```python
from build123d import *

# Parameters (mm, degrees)
BOSS_EXTRUDE1_DEPTH = 4.7625
SKETCH3_W           = 66.200858932
SKETCH3_H           = 5.079818348
BOSS_EXTRUDE2_DEPTH = 31.75
SKETCH4_W           = 28.999942
SKETCH4_H           = 12.9999994
CUT_EXTRUDE1_DEPTH  = 4.7625
SKETCH5_R           = 6.4999997
CUT_EXTRUDE2_DEPTH  = 4.7625
SKETCH6_R           = 3.175
CUT_EXTRUDE3_DEPTH  = 7.3025


with BuildPart() as part:
    # Sketch1 → Boss-Extrude1 (new body)
    with BuildSketch(Plane.XY):
        Polygon((30.222809818, 36.11360466), (25.142809818, 48.349181892), (-47.247190182, 48.349181892), (-52.327190182, 36.11360466), (-52.327190182, -53.715240876), (-47.247190182, -65.950818108), (25.142809818, -65.950818108), (30.222809818, -53.715240876), align=None)
    extrude(amount=BOSS_EXTRUDE1_DEPTH)

    # Sketch3 → Boss-Extrude2 (add)
    with BuildSketch(Plane.XY.offset(4.7625)):
        with Locations((-11.098760716, 45.809272718)):
            Rectangle(SKETCH3_W, SKETCH3_H)
        with Locations((-11.098760716, -63.410908934)):
            Rectangle(SKETCH3_W, SKETCH3_H)
    extrude(amount=BOSS_EXTRUDE2_DEPTH)

    # Sketch4 → Cut-Extrude1 (cut)
    with BuildSketch(Plane(origin=(0, 0, 0), x_dir=(-1, 0, 0), z_dir=(0, 0, -1))):
        with Locations((11.052190182, -27.850818108)):
            Rectangle(SKETCH4_W, SKETCH4_H)
    extrude(amount=-CUT_EXTRUDE1_DEPTH, mode=Mode.SUBTRACT)

    # Sketch5 → Cut-Extrude2 (cut)
    with BuildSketch(Plane(origin=(0, 0, 0), x_dir=(-1, 0, 0), z_dir=(0, 0, -1))):
        with Locations((11.052190182, 10.249181892)):
            Circle(SKETCH5_R)
    extrude(amount=-CUT_EXTRUDE2_DEPTH, mode=Mode.SUBTRACT)

    # Sketch6 → Cut-Extrude3 (cut)
    with BuildSketch(Plane.XZ.offset(65.950818108)):
        with Locations((-11.052190182, 20.6375)):
            Circle(SKETCH6_R)
    extrude(amount=-CUT_EXTRUDE3_DEPTH, mode=Mode.SUBTRACT)


solid = part.part
```
Verification items for the finished model (mm, model axes). A direction names the side the tool comes from. Give positions to 0.01 mm unless a question says otherwise; leave off trailing zeros. Loops run counter-clockwise (first coordinate to the right, second up) from the corner with the lowest first, then second, coordinate; pieces in that order, holes last.
1. Section check B-B, the plane z = 10. Enter the section's corners in (x, y).
2. Set-up check for faces 1 (the flat face through (-12, -60.871, 24)), 2 (the flat face through (-11, -34.351, 2)), 3 (the flat face through (22.002, -63, 20)), 4 (the flat face through (-44.199, -63, 20)): record each of +Z, -Z, +X, -X, +Y, -Y from which the full face is reachable in a straight line by a thin tool's end or side.
3. Go/stop test with flat-tipped pins: pin 1 Ø15 at (x, y) = (-11.05, 10.25) entering from +Z; pin 2 Ø2.5 at (y, z) = (46, 27) entering from +X; pin 3 Ø1.5 at (y, z) = (46, 25.5) entering from -X. Record where each tip stops, or that it passes through.
4. Thickness scan on line 1 (Y direction, x = 17.5, z = 20); line 2 (X direction, y = -28, z = 2); line 3 (Z direction, x = -45, y = -50.5). Record the ranges inside material, lowest first.
5. Section check D-D, the plane x = 8. Enter the section's corners in (y, z).
6. Section check A-A, the plane y = -27. Enter the section's corners in (x, z), then the cut area to 3 significant figures.
7. Mould release check, pull along Z, two halves, no side actions. Record for faces 5 (the flat face through (-12, 43.269, 20)), 6 (the flat face through (-12, -8, 0)), 7 (the cylindrical face through (-14.224, -63.446, 20.777)), 8 (the flat face through (-12, 46, 36.512)): released by +Z, released by -Z, zero draft, split by the parting line, or undercut.
8. Section check C-C, the plane z = 22.5. Enter the section's corners in (x, y), then the cut area to 3 significant figures.
Geometry says:
1. outline: (-44.2, -65.95) - (22, -65.95) - (22, -60.87) - (-44.2, -60.87) - close; (-44.2, 43.27) - (22, 43.27) - (22, 48.35) - (-44.2, 48.35) - close
2. face 1: +Z, +X, -X
2. face 2: +Z, -Z
2. face 3: +Z, +X, +Y, -Y
2. face 4: +Z, -X, +Y, -Y
3. pin 1: stops at z = 4.76
3. pin 2: stops at x = 22
3. pin 3: stops at x = -44.2
4. line 1: y = -65.95 to -60.87, 43.27 to 48.35
4. line 2: x = -52.33 to -25.55, 3.45 to 30.22
4. line 3: z = 0 to 4.76
5. outline: (-65.95, 0) - (48.35, 0) - (48.35, 36.51) - (43.27, 36.51) - (43.27, 4.76) - (-60.87, 4.76) - (-60.87, 36.51) - (-65.95, 36.51) - close
6. outline: (-52.33, 0) - (-25.55, 0) - (-25.55, 4.76) - (-52.33, 4.76) - close; (3.45, 0) - (30.22, 0) - (30.22, 4.76) - (3.45, 4.76) - close
6. area: 255 mm2
7. face 5: zero draft
7. face 6: released by -Z
7. face 7: undercut
7. face 8: released by +Z
8. outline: (-44.2, -65.95) - (-13.62, -65.95) - (-13.62, -60.87) - (-44.2, -60.87) - close; (-44.2, 43.27) - (22, 43.27) - (22, 48.35) - (-44.2, 48.35) - close; (-8.48, -65.95) - (22, -65.95) - (22, -60.87) - (-8.48, -60.87) - close
8. area: 646 mm2
